Geometry: final body of the model. Coordinates: model frame, mm. Give positions to 0.01 mm unless a question says otherwise; leave off trailing zeros. Order: outer loops, then holes, each group sorted by start corner. A loop starts at its lowest first (then second) coordinate and runs counter-clockwise, first axis right, second up. Notation, with made-up numbers: (85.25, 89) - (93.25, 89) arc R25 ccw to (93.25, 108) - close; hole circle Ø10 at (25.5, 38). An arc over 180 degrees is marked (long way). One line per item, written item: value.
Autodesk Inventor part; units mm, degrees
ref_plane "Work Plane1" through (0, 120, 0) normal (0, 1, 0) x (-1, 0, 0)
ref_plane "YZ Plane" through (0, 0, 0) normal (1, 0, 0) x (0, 1, 0)
ref_plane "XY Plane" through (0, 0, 0) normal (0, 0, 1) x (1, 0, 0)
sketch "Sketch1" plane through (0, 0, 0) normal (0, 0, 1) x (1, 0, 0)
  line L0 (-10, 135) -> (-10, 230)
  line L1 (-10, 230) -> (-100, 230)
  line L2 (-100, 230) -> (-100, 240)
  line L3 (-100, 240) -> (100, 240)
  line L4 (100, 240) -> (100, 230)
  line L5 (100, 230) -> (10, 230)
  line L6 (10, 230) -> (10, 135)
  line L7 (10, 135) -> (100, 135)
  line L8 (100, 135) -> (100, 105)
  line L9 (100, 105) -> (10, 105)
  line L10 (10, 105) -> (10, 10)
  line L11 (10, 10) -> (100, 10)
  line L12 (100, 10) -> (100, 0)
  line L13 (100, 0) -> (-100, 0)
  line L14 (-100, 0) -> (-100, 10)
  line L15 (-100, 10) -> (-10, 10)
  line L16 (-10, 10) -> (-10, 105)
  line L17 (-10, 105) -> (-100, 105)
  line L18 (-100, 105) -> (-100, 135)
  line L19 (-100, 135) -> (-10, 135)
  line L20 (0, 0) -> (0, 240) construction
  dimension "d0" = 10
  dimension "d1" = 200
  dimension "d2" = 20
  dimension "d3" = 30
  dimension "d4" = 10
  dimension "d5" = 95
  dimension "d6" = 95
extrude "Extrusion1" add sketch "Sketch1" against normal blind 8
sketch "Sketch2" plane through (0, 0, 0) normal (0, 0, 1) x (1, 0, 0)
  line L0 (-10, 135) -> (-100, 135)
  line L1 (-100, 0) -> (100, 0)
  line L2 (-100, 240) -> (-100, 230)
  line L3 (-100, 10) -> (-100, 0)
  point P0 (0, 0)
  point P1 (-67.5, 120)
  point P2 (-22.5, 120)
  point P3 (22.5, 120)
  point P4 (67.5, 120)
  point P5 (0, 0)
  point P6 (-67.5, 235)
  point P7 (67.5, 235)
  point P8 (67.5, 5)
  point P9 (-67.5, 5)
  point P10 (-100, 235)
  point P11 (-100, 5)
  point P12 (0, 0)
  dimension "d9" = 15
  dimension "d10" = 67.5
  dimension "d11" = 45
  dimension "d12" = 45
  dimension "d13" = 45
  dimension "d14" = 67.5
  dimension "d15" = 135
hole "Hole1" at (-67.5, 120, 0) at (-22.5, 120, 0) at (22.5, 120, 0) at (67.5, 120, 0) at (-67.5, 235, 0) at (67.5, 235, 0) at (67.5, 5, 0) at (-67.5, 5, 0) direction (0, 0, -1) diameter 5 depth 8
sketch "Sketch3" plane through (-100, 0, 0) normal (0, -1, 0) x (1, 0, 0)
  line L0 (0, 0) -> (200, 0)
  line L1 (200, -8) -> (0, -8)
  point P0 (100, 0)
  point P1 (10, -4)
  point P2 (55, -4)
  point P3 (145, -4)
  point P4 (190, -4)
  point P5 (100, 0)
  point P6 (100, -4)
  point P7 (100, 0)
  dimension "d23" = 4
  dimension "d24" = 45
  dimension "d25" = 90
  dimension "d26" = 90
  dimension "d27" = 45
hole "Hole2" at (-90, 0, -4) at (-45, 0, -4) at (45, 0, -4) at (90, 0, -4) at (0, 0, -4) direction (0, 1, 0) diameter 5 depth 10
ref_plane "Work Plane1" through (0, 120, 0) normal (0, 1, 0) x (-1, 0, 0)
mirror "Mirror1" about plane through (0, 120, 0) normal (0, 1, 0) of "Hole2"
sketch "Sketch4" plane through (-100, 105, 0) normal (0, -1, 0) x (1, 0, 0)
  circle A0 centre (100, -4) radius 2.5
  line L0 (0, -8) -> (90, -8)
  point P0 (100, 0)
  point P1 (10, -4)
  point P2 (55, -4)
  point P3 (145, -4)
  point P4 (190, -4)
  dimension "d36" = 4
  dimension "d37" = 180
  dimension "d38" = 90
  dimension "d39" = 45
  dimension "d48" = 45
hole "Hole3" at (-90, 105, -4) at (-45, 105, -4) at (45, 105, -4) at (90, 105, -4) direction (0, 1, 0) diameter 5 depth 30
equation "\"d6\" = d5"
properties part number "02" material "Aluminum 6061"
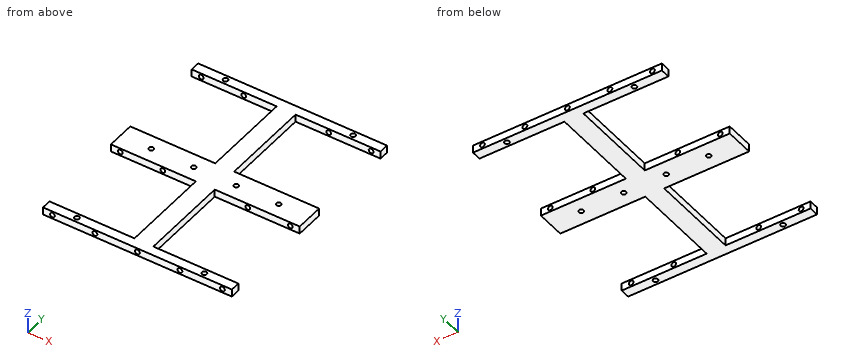
1) Section B-B, the plane y = 85.5. Return loops of the section in (x, z), then the cut area to 3 significant figures.
Answers below:
outline: (-10, -8) - (10, -8) - (10, 0) - (-10, 0) - close
area: 160 mm^2
2) Section A-A, the plane z = -4.5. Count the separate pieces of the cut face and the enclosed holes in it, then the cut area to 3 significant figures.
Answers below:
separate pieces: 13
enclosed holes: 8
area: 12,600 mm^2
3) First-contact query: pin 1 (8 mm diameter, centred on x = 67.5, y = 120, fed in from +Z); pin 2 (1.5 mm diameter, centred on y = 151, z = -2, fed in from -X); pin 3 (2 mm diameter, centred on y = 210, z = -5, fed in from +X). Flat tips, straight axial feed; report the tip coordinate or a pass-through.
Answers below:
pin 1: z = 0
pin 2: x = -10
pin 3: x = 10
4) Material intervals for line 1 along X through (y, z) = (125.75, -4); line 2 along Y through (x, z) = (53.5, -0.25); line 3 along Y through (x, z) = (-67.5, -3.5), sorted ascending.
Answers below:
line 1: -100 to -92.5, -87.5 to -47.5, -42.5 to 42.5, 47.5 to 87.5, 92.5 to 100
line 2: 0 to 10, 105 to 135, 230 to 240
line 3: 0 to 2.5, 7.5 to 10, 105 to 117.5, 122.5 to 135, 230 to 232.5, 237.5 to 240
